Could you check a few things on this drawing? It's one solid part, dimensions in mm from its lowest x, y, z. A direction names the side the tool comes from. Coordinates: 2 decimals unless noted, no trailing zeros. Order: outer loops, then holes, each group sorted by start corner. A loop starts at its lowest first (then second) coordinate and runs counter-clockwise, first axis right, second up. Notation, with made-up numbers: (-28, 43) - (24, 43) arc R22 ccw to (24, 52) - close; hole circle Ø1 at (69.25, 34). An arc over 180 degrees is marked (long way). Answer in a Markdown table with one row per item. Add a question column.
Item 1: If I drill on line 1 along Y through (x, z) = (33, 4.95); line 2 along Z through (x, y) = (34, 8); line 3 along Y through (x, z) = (30.5, 1), over which ranges is the centre line in solid material (lowest first)? Write a range as from..to.
Item 2: I want a section at C-C (y = 3.5). Please give me the cut outline in (x, z), plus the area to 3 significant figures.
Item 3: Will these pins go through, and if not, where does the flat tip stop? pin 1 Ø2 at (y, z) = (11.5, 3) entering from -X; pin 2 Ø12 at (x, y) = (6.5, 13.5) entering from +Z; pin 3 Ø8 at (x, y) = (17.5, 8.5) entering from -Z.
Item 4: I want a section at B-B (z = 0.6). Please give me the cut outline in (x, y), plus the area to 3 significant figures.
Item 5: I want a section at A-A (x = 19.5). Please give me the cut outline in (y, z), plus the area to 3 significant figures.
Item 6: On a 3-axis mill with a long thin cutter (end or side, diameter ignored), from which of +Z, -Z, +X, -X, +Y, -Y can I reach the whole of each face in a straight line? I mean the marked faces 1 and 2. Say none if no direction works.
Item 7: I want a section at D-D (z = 2.45). Please give me the cut outline in (x, y), plus the area to 3 significant figures.
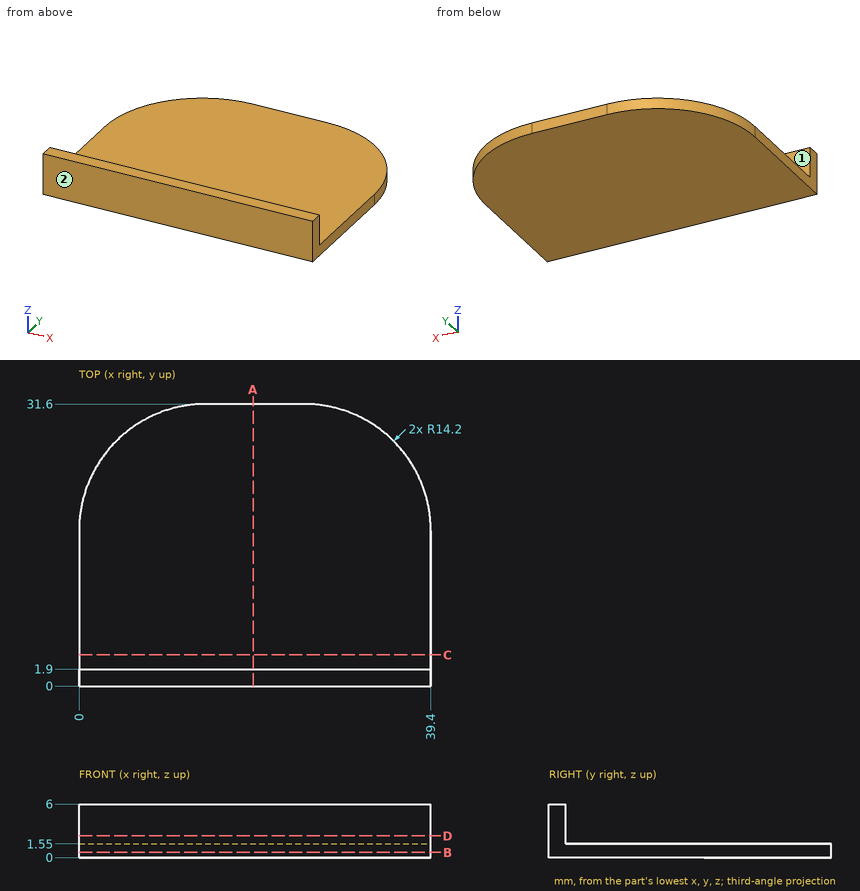
Values follow:
| question | item | result |
|---|---|---|
| 1 | line 1 | y = 0..1.9 |
| 1 | line 2 | z = 0..1.55 |
| 1 | line 3 | y = 0..30.57 |
| 2 | outline | (0, 0) - (39.4, 0) - (39.4, 1.55) - (0, 1.55) - close |
| 2 | area | 61.1 mm^2 |
| 3 | pin 1 | passes through |
| 3 | pin 2 | stops at z = 1.55 |
| 3 | pin 3 | stops at z = 0 |
| 4 | outline | (0, 0) - (39.4, 0) - (39.4, 17.4) arc R14.2 ccw to (25.2, 31.6) - (14.2, 31.6) arc R14.2 ccw to (0, 17.4) - close |
| 4 | area | 1,160 mm^2 |
| 5 | outline | (0, 0) - (31.6, 0) - (31.6, 1.55) - (1.9, 1.55) - (1.9, 6) - (0, 6) - close |
| 5 | area | 57.4 mm^2 |
| 6 | face 1 | +Z, +X, -X, +Y |
| 6 | face 2 | +Z, -Z, +X, -X, -Y |
| 7 | outline | (0, 0) - (39.4, 0) - (39.4, 1.9) - (0, 1.9) - close |
| 7 | area | 74.9 mm^2 |
